The model under review builds one solid part; all positions refer to its coordinate system, in mm. A direction names the side the tool comes from. Coordinates: 2 decimals unless noted, no trailing zeros. Write each loop counter-clockwise with the first axis right and the second up, starting at its lowest first coordinate (ties: lowest second). Pieces come first, ordered by that corner, then holes.
```python
from build123d import *

# Parameters (mm, degrees)
SKETCH1_W            = 16
SKETCH1_H            = 30
BOSS_EXTRUDE1_DEPTH  = 24
SKETCH2_W            = 2
SKETCH2_H            = 30
CUT_EXTRUDE1_DEPTH   = 2
M4_CLEARANCE_HOLE1_D = 4.5


with BuildPart() as part:
    # Sketch1 → Boss-Extrude1 (new body)
    with BuildSketch(Plane(origin=(0, 0, 0), x_dir=(0, 0, -1), z_dir=(1, 0, 0))):
        with Locations((-8, 15)):
            Rectangle(SKETCH1_W, SKETCH1_H)
    extrude(amount=BOSS_EXTRUDE1_DEPTH)

    # Sketch2 → Cut-Extrude1 (cut)
    with BuildSketch(Plane.ZY):
        with Locations((1, 15)):
            Rectangle(SKETCH2_W, SKETCH2_H)
    extrude(amount=-CUT_EXTRUDE1_DEPTH, mode=Mode.SUBTRACT)

    # M4 Clearance Hole1 (through all)
    with Locations(Plane(origin=(24, 0, 0), x_dir=(0, 0, -1), z_dir=(1, 0, 0))):
        with Locations((-9, 15)):
            Hole(M4_CLEARANCE_HOLE1_D / 2)


solid = part.part
```
Item 1: Take a section at B-B, the plane z = 9. Write out the cut boundary in (x, y), plus the area to 3 significant figures.
Solved:
outline: (0, 0) - (24, 0) - (24, 12.75) - (0, 12.75) - close; (0, 17.25) - (24, 17.25) - (24, 30) - (0, 30) - close
area: 612 mm2
Item 2: Mouldability with a two-part tool opening along Y and no side actions: class faces 1 (the face through (11.832, 12.804, 8.512)), 2 (the face through (12, 0, 8)), 3 (the face through (0, 15, 6)) as pulls with the +Y half, pulls with the -Y half, needs draft (parallel to the pull), parting line crosses it, or undercut.
Solved:
face 1: undercut
face 2: pulls with the -Y half
face 3: needs draft
Item 3: Take a section at A-A, the plane y = 15. Write out the cut boundary in (x, z).
Solved:
outline: (0, 2) - (2, 2) - (2, 0) - (24, 0) - (24, 6.75) - (0, 6.75) - close; (0, 11.25) - (24, 11.25) - (24, 16) - (0, 16) - close
Item 4: For pin 1 (1 mm diameter, centred on x = 1, y = 9, fed in from -Z); pin 2 (0.6 mm diameter, centred on y = 12, z = 1, fed in from -X); pin 3 (3.5 mm diameter, centred on y = 15, z = 9, fed in from +X), all flat-tipped, find the tip position at first contact; note any pin that passes through.
Solved:
pin 1: stops at z = 2
pin 2: stops at x = 2
pin 3: passes through
Item 5: Machinability: for faces 4 (the face through (2, 15, 1)), 5 (the face through (12, 15, 16)), which of the approach directions +Z, -Z, +X, -X, +Y, -Y give a long, thin tool a straight path to every point of the face, cutting with its end or side? Answer none if there is none.
Solved:
face 4: -Z, -X, +Y, -Y
face 5: +Z, +X, -X, +Y, -Y
Item 6: Take a section at C-C, the plane x = 5.75. Write out the cut boundary in (y, z), plus the area to 3 significant figures.
Solved:
outline: (0, 0) - (30, 0) - (30, 16) - (0, 16) - close; hole circle Ø4.5 at (15, 9)
area: 464 mm2
Item 7: To check wall thickness, follow line 1 along Y through (x, z) = (9, 9); line 2 along Z through (x, y) = (13, 14.5); line 3 along X through (y, z) = (27.75, 1.75). State the ranges of each line that lie inside material, in increasing order.
Solved:
line 1: y = 0 to 12.75, 17.25 to 30
line 2: z = 0 to 6.81, 11.19 to 16
line 3: x = 2 to 24
